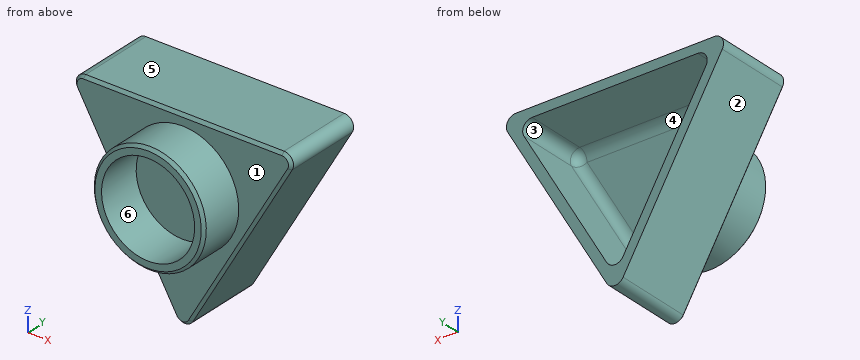
```python
from build123d import *

# Parameters (mm, degrees)
BOSS_EXTRUDE1_DEPTH = 21.42998
SHELL1_T            = -2.54
SKETCH3_R           = 15.08125
BOSS_EXTRUDE2_DEPTH = 11.90498
FILLET1_R           = 2.54
FILLET2_R           = 2.54
FILLET3_R           = 2.54
CHAMFER2_SIZE       = 0.762
SKETCH5_R           = 12.54125
CUT_EXTRUDE1_DEPTH  = 11.90498
CHAMFER3_SIZE       = 0.762


with BuildPart() as part:
    # Sketch1 → Boss-Extrude1 (new body)
    with BuildSketch(Plane(origin=(0, 0, 0), x_dir=(1, 0, 0), z_dir=(0, 1, 0))):
        Polygon((0, 35.91687), (31.104921844, -17.958435), (-31.104921844, -17.958435), align=None)
    extrude(amount=BOSS_EXTRUDE1_DEPTH)

    # Shell1
    shell1_openings = [part.faces().sort_by_distance(p)[0] for p in [
        (0, 21.42998, 0),
    ]]
    offset(amount=SHELL1_T, openings=shell1_openings, kind=Kind.INTERSECTION)

    # Sketch3 → Boss-Extrude2 (add)
    with BuildSketch(Plane.XZ):
        with Locations(Location((0, 0, 0), (0, 0, 90))):
            Circle(SKETCH3_R)
    extrude(amount=BOSS_EXTRUDE2_DEPTH)

    # Fillet1
    fillet1_edges = [part.edges().sort_by_distance(p)[0] for p in [
        (0, 10.71499, -35.91687),
        (31.104921844, 10.71499, 17.958435),
        (-31.104921844, 10.71499, 17.958435),
    ]]
    fillet(fillet1_edges, radius=FILLET1_R)

    # Fillet2
    fillet2_edges = [part.edges().sort_by_distance(p)[0] for p in [
        (0, 11.98499, -30.83687),
        (-26.705512793, 11.98499, 15.418435),
        (26.705512793, 11.98499, 15.418435),
    ]]
    fillet(fillet2_edges, radius=FILLET2_R)

    # Fillet3
    fillet3_edges = [part.edges().sort_by_distance(p)[0] for p in [
        (13.352756397, 2.54, -7.7092175),
        (-13.352756397, 2.54, -7.7092175),
        (0, 2.54, 15.418435),
        (-24.505808268, 2.54, 14.148435),
        (24.505808268, 2.54, 14.148435),
        (0, 2.54, -28.29687),
    ]]
    fillet(fillet3_edges, radius=FILLET3_R)

    # Chamfer2
    chamfer2_edges = [part.edges().sort_by_distance(p)[0] for p in [
        (-15.552460922, 0, -8.9792175),
        (15.552460922, 0, -8.9792175),
        (0, 0, 17.958435),
        (-28.905217319, 0, 16.688435),
        (28.905217319, 0, 16.688435),
        (0, 0, -33.37687),
    ]]
    chamfer(chamfer2_edges, length=CHAMFER2_SIZE)

    # Sketch5 → Cut-Extrude1 (cut)
    with BuildSketch(Plane.XZ.offset(11.90498)):
        with Locations(Location((0, 0, 0), (0, 0, 270))):
            Circle(SKETCH5_R)
    extrude(amount=-CUT_EXTRUDE1_DEPTH, mode=Mode.SUBTRACT)

    # Chamfer3
    chamfer3_edges = [part.edges().sort_by_distance(p)[0] for p in [
        (0, -11.90498, -15.08125),
    ]]
    chamfer(chamfer3_edges, length=CHAMFER3_SIZE)


solid = part.part
```
Design review of the part built by this model. Coordinates are the model's own, in mm. Face numbers are marked on the shaded views. A direction names the side the tool comes from. Round coordinates to 2 decimals unless told otherwise and drop trailing zeros. Write each loop counter-clockwise with the first axis right and the second up, starting at its lowest first coordinate (ties: lowest second). Pieces come first, ordered by that corner, then holes. Notation, with made-up numbers: (-25, 4.25) -> (5, 4.25) arc R32 ccw to (5, 41.25) -> close; hole circle Ø11 at (-16.5, 56). An arc over 180 degrees is marked (long way). Write item = value, one per line. Start each with the question number.
1) Clearance check with flat-ended pins moving along their axes: pin 1 (12 mm diameter, centred on x = -16, y = 4.5, fed in from -Z); pin 2 (1.5 mm diameter, centred on x = -18, y = 0.5, fed in from -Z); pin 3 (20 mm diameter, centred on x = 0, z = 0, fed in from -Y). State where each tip first meets the part, or that it passes through.
2) Take a section at A-A, the plane y = 8.5. State the section outline as (x, z) points, plus the area to 3 significant figures.
3) Tool access review of the marked faces 4, 5 and 6: name each direction out of +Z, -Z, +X, -X, +Y, -Y from which nothing blocks a thin tool from reaching the whole face with its end or side.
4) Wall thickness on probe 1 along X at (y, z) = (-7, 0); probe 2 along Y at (x, z) = (-6.5, 2); probe 3 along Y at (x, z) = (11, -13): over which ranges is each line inside the solid? List them lowest first. Write a range as from..to.
5) Take a section at B-B, the plane y = -1. State the section outline as (x, z) points.
6) Mouldability with a two-part tool opening along X and no side actions: class the marked faces 1, 2 and 3 as +X half, -X half, draft (parallel to the pull), parting line (faces both ways), or undercut.
Results list:
q1.pin_1 = -18.6
q1.pin_2 = -5.96
q1.pin_3 = 0
q2.outline = (-28.91, 14.15) -> (-2.2, -32.11) arc R2.54 ccw to (2.2, -32.11) -> (28.91, 14.15) arc R2.54 ccw to (26.71, 17.96) -> (-26.71, 17.96) arc R2.54 ccw to start; hole (-24.51, 11.61) -> (-2.2, -27.03) arc R2.54 ccw to (2.2, -27.03) -> (24.51, 11.61) arc R2.54 ccw to (22.31, 15.42) -> (-22.31, 15.42) arc R2.54 ccw to start
q2.area = 441 mm²
q3.face_4 = +Y
q3.face_5 = +Z, +X, -X, +Y, -Y
q3.face_6 = -Y
q4.probe_1 = -15.08..-12.54, 12.54..15.08
q4.probe_2 = 0..2.54
q4.probe_3 = 0..21.43
q5.outline = circle Ø30.16 at (0, 0); hole circle Ø25.08 at (0, 0)
q6.face_1 = draft
q6.face_2 = -X half
q6.face_3 = undercut
